Autodesk Inventor part; units mm, degrees
ref_plane "YZ Plane" through (0, 0, 0) normal (1, 0, 0) x (0, 1, 0)
ref_plane "XZ Plane" through (0, 0, 0) normal (0, 1, 0) x (-1, 0, 0)
ref_plane "XY Plane" through (0, 0, 0) normal (0, 0, 1) x (1, 0, 0)
sketch "Sketch1" plane through (0, 0, 0) normal (0, 1, 0) x (-1, 0, 0)
  line L0 (101.6, 0) -> (812.8, 0)
  line L1 (914.4, 101.6) -> (914.4, 508)
  line L2 (812.8, 609.6) -> (101.6, 609.6)
  line L3 (0, 508) -> (0, 101.6)
  arc A0 (101.6, 609.6) -> (0, 508) centre (101.6, 508) ccw
  arc A1 (0, 101.6) -> (101.6, 0) centre (101.6, 101.6) ccw
  arc A2 (812.8, 0) -> (914.4, 101.6) centre (812.8, 101.6) ccw
  arc A3 (914.4, 508) -> (812.8, 609.6) centre (812.8, 508) ccw
  point P0 (0, 0)
  point P1 (914.4, 609.6)
  point P2 (914.4, 0)
  point P3 (0, 609.6)
  dimension "d0" = 914.4
  dimension "d1" = 609.6
  dimension "d9" = 101.6
extrude "Extrusion1" add sketch "Sketch1" along normal blind 50.8
sketch "Sketch3" plane through (0, 50.8, 0) normal (0, 1, 0) x (1, 0, 0)
  line L0 (0, -508) -> (0, -101.6)
  arc A0 (0, -101.6) -> (-101.6, 0) centre (-101.6, -101.6) ccw
  line L1 (-101.6, 0) -> (-812.8, 0)
  arc A1 (-812.8, 0) -> (-914.4, -101.6) centre (-812.8, -101.6) ccw
  line L2 (-914.4, -101.6) -> (-914.4, -508)
  arc A2 (-914.4, -508) -> (-812.8, -609.6) centre (-812.8, -508) ccw
  line L3 (-812.8, -609.6) -> (-101.6, -609.6)
  arc A3 (-101.6, -609.6) -> (0, -508) centre (-101.6, -508) ccw
  line L4 (-812.8, -50.8) -> (-101.6, -50.8)
  arc A4 (-50.8, -101.6) -> (-101.6, -50.8) centre (-101.6, -101.6) ccw
  line L5 (-50.8, -101.6) -> (-50.8, -508)
  arc A5 (-101.6, -558.8) -> (-50.8, -508) centre (-101.6, -508) ccw
  line L6 (-101.6, -558.8) -> (-812.8, -558.8)
  arc A6 (-863.6, -508) -> (-812.8, -558.8) centre (-812.8, -508) ccw
  line L7 (-863.6, -508) -> (-863.6, -101.6)
  arc A7 (-812.8, -50.8) -> (-863.6, -101.6) centre (-812.8, -101.6) ccw
  point P0 (0, 0)
  dimension "d10" = 50.8
extrude "Extrusion3" add sketch "Sketch3" along normal blind 762
sketch "Sketch10" plane through (0, 0, 508) normal (1, 0, 0) x (0, 0, -1)
  circle A0 centre (50.8, 152.4) radius 22.5
  circle A1 centre (152.4, 152.4) radius 22.5
  circle A2 centre (254, 152.4) radius 22.5
  circle A3 centre (355.6, 152.4) radius 22.5
  line L0 (0, 0) -> (0, 812.8)
  line L1 (0, 0) -> (406.4, 0)
  circle A4 centre (50.8, 304.8) radius 22.5
  circle A5 centre (152.4, 304.8) radius 22.5
  circle A6 centre (254, 304.8) radius 22.5
  circle A7 centre (355.6, 304.8) radius 22.5
  dimension "d56" = 45
  dimension "d57" = 45
  dimension "d58" = 45
  dimension "d59" = 45
  dimension "d60" = 50.8
  dimension "d61" = 101.6
  dimension "d62" = 101.6
  dimension "d63" = 101.6
  dimension "d64" = 152.4
  dimension "d67" = 45
  dimension "d68" = 45
  dimension "d69" = 45
  dimension "d70" = 45
  dimension "d71" = 152.4
extrude "Extrusion4" cut sketch "Sketch10" against normal through all
properties part number "pullbox"
For this review, take the finished solid that the model builds, in its own axes (mm). A direction names the side the tool comes from. Round coordinates to 2 decimals unless told otherwise and drop trailing zeros. Write each loop counter-clockwise with the first axis right and the second up, starting at its lowest first coordinate (ties: lowest second). Pieces come first, ordered by that corner, then holes. Notation, with made-up numbers: (51, 51.5) - (58, 51.5) arc R15 ccw to (58, 75.5) - close; hole circle Ø8 at (55, -25). An arc over 180 degrees is marked (long way). Use CSV: the item, a comma, the result in double quotes.
1) For faces 5 (the flat face through (-863.6, 426, 308)), 6 (the cylindrical face through (-25.04, 153.39, 174.88)), list the 3-axis set-ups (+Z, -Z, +X, -X, +Y, -Y) from which the entire face can be reached by the end or side of a thin tool; tool diameter is ignored.
Conclusion:
face 5,"+Y"
face 6,"+X, -X"
2) Add section D-D on y = 304.8. Count the separate pieces of the cut face and the enclosed holes in it, and give its area (3 significant figures).
Conclusion:
separate pieces,"8"
enclosed holes,"0"
area,"120,000 mm^2"
3) Add section B-B on y = 395.5. Write out the cut boundary in (x, z).
Conclusion:
outline,"(-914.4, 101.6) arc R101.6 ccw to (-812.8, 0) - (-101.6, 0) arc R101.6 ccw to (0, 101.6) - (0, 508) arc R101.6 ccw to (-101.6, 609.6) - (-812.8, 609.6) arc R101.6 ccw to (-914.4, 508) - close; hole (-863.6, 101.6) arc R50.8 ccw to (-812.8, 50.8) - (-101.6, 50.8) arc R50.8 ccw to (-50.8, 101.6) - (-50.8, 508) arc R50.8 ccw to (-101.6, 558.8) - (-812.8, 558.8) arc R50.8 ccw to (-863.6, 508) - close"
4) Clearance check with a flat-ended pin moving along its axis: pin 1 Ø8 at (x, z) = (-147.5, 511) entering from +Y. State where the tip first meets the part, or that it passes through.
Conclusion:
pin 1,"stops at y = 50.8"
5) Add section C-C on x = -495. Write out the cut boundary in (y, z), and give its area (3 significant figures).
Conclusion:
outline,"(0, 0) - (812.8, 0) - (812.8, 50.8) - (50.8, 50.8) - (50.8, 558.8) - (812.8, 558.8) - (812.8, 609.6) - (0, 609.6) - close"
area,"108,000 mm^2"
6) Wall thickness on line 1 along Y through (x, z) = (-24, 152); line 2 along X through (y, z) = (420.5, 96.5); line 3 along X through (y, z) = (591, 504): over which ranges is each line inside the solid? List them lowest first. Write a range as from..to.
Conclusion:
line 1,"y = 0..129.9, 174.9..282.3, 327.3..812.8"
line 2,"x = -914.27..-863.34, -51.06..-0.13"
line 3,"x = -914.4..-863.6, -50.8..0"
7) The part is to be moulded in two halves that separate along Y. For faces 1 (the cylindrical face through (-25.04, 305.79, 378.08)), 2 (the cylindrical face through (-28.972, 400.71, 579.048)), 3 (the cylindrical face through (-888.64, 153.39, 174.88)), 4 (the flat face through (-493, 812.8, 574)), say which applies: pulls with the +Y half, pulls with the -Y half, needs draft (parallel to the pull), parting line crosses it, or undercut.
Conclusion:
face 1,"undercut"
face 2,"needs draft"
face 3,"undercut"
face 4,"pulls with the +Y half"
8) Add section A-A on z = 457.2. Write out the cut boundary in (x, y), and give its area (3 significant figures).
Conclusion:
outline,"(-914.4, 0) - (0, 0) - (0, 129.9) - (-50.8, 129.9) - (-50.8, 50.8) - (-863.6, 50.8) - (-863.6, 129.9) - (-914.4, 129.9) - close; (-914.4, 174.9) - (-863.6, 174.9) - (-863.6, 282.3) - (-914.4, 282.3) - close; (-914.4, 327.3) - (-863.6, 327.3) - (-863.6, 812.8) - (-914.4, 812.8) - close; (-50.8, 174.9) - (0, 174.9) - (0, 282.3) - (-50.8, 282.3) - close; (-50.8, 327.3) - (0, 327.3) - (0, 812.8) - (-50.8, 812.8) - close"
area,"115,000 mm^2"
